```python
from build123d import *

# Parameters (mm, degrees)
F1_DEPTH = 10
F2_D     = 12
F2_DEPTH = 30


with BuildPart() as f1:
    # F0 (on Front) → F1 (new body)
    with BuildSketch(Plane.XZ):
        with BuildLine():
            ThreePointArc((0, -40), (8.838835, -36.338835), (12.5, -27.5))
            Line((12.5, -27.5), (12.5, 27.5))
            ThreePointArc((12.5, 27.5), (8.838835, 36.338835), (0, 40))
            ThreePointArc((0, 40), (-8.838835, 36.338835), (-12.5, 27.5))
            Line((-12.5, 27.5), (-12.5, -27.5))
            ThreePointArc((-12.5, -27.5), (-8.838835, -36.338835), (0, -40))
        make_face()
    extrude(amount=F1_DEPTH)

    # F2
    with Locations(Plane(origin=(0, 0, 0), x_dir=(1, 0, 0), z_dir=(0, 1, 0))):
        with Locations((0, 27.5), (0, -27.5)):
            Hole(F2_D / 2, depth=F2_DEPTH)


solid = f1.part
```
Could you check a few things on this model? Use its own coordinates, in mm. Coordinates: 2 decimals unless noted, no trailing zeros. Loops run counter-clockwise (first coordinate to the right, second up) from the corner with the lowest first, then second, coordinate; pieces in that order, holes last. Notation, with made-up numbers: M -28.5,57.5 L 25.5,57.5 A11 cw 25.5,69.5 Z; hole C 86,83.5 d4. An arc over 180 degrees is marked long. Put each result on its own line as item: value. Start each with the question number.
(1) I need wall thicknesses on line 1 (Z direction, x = 0, y = -3.25); line 2 (X direction, y = -6, z = -27.5); line 3 (Z direction, x = -1.5, y = -4.25). Which ranges of each line are inside material? Lowest first, please. Write a range as from..to.
(2) Suppose I cut it at A-A on z = -31.5. Please give me the cut outline in (x, y).
(3) Suppose I cut it at B-B on y = -8.5. Please give me the cut outline in (x, z), then the cut area to 3 significant figures.
(4) Will this pin go through, and if not, where does the flat tip stop? P1, Ø9.5, axis at x = 0, z = -27.5, coming from the +Y side.
(5) Suppose I cut it at C-C on x = -7. Please give me the cut outline in (y, z), then the cut area to 3 significant figures.
(6) Thinking about a two-plate mould opening in Z: for faces 1 (the face through (-12.5, -5, 0)), 2 (the face through (1.301, -5.07, -21.643)), which applies, pulls with the +Z half, pulls with the -Z half, needs draft (parallel to the pull), parting line crosses it, or undercut?
Solutions:
1. line 1: z = -40..-33.5, -21.5..21.5, 33.5..40
1. line 2: x = -12.5..-6, 6..12.5
1. line 3: z = -39.91..-33.31, -21.69..21.69, 33.31..39.91
2. outline: M -11.84,-10 L -4.47,-10 L -4.47,0 L -11.84,0 Z; M 4.47,-10 L 11.84,-10 L 11.84,0 L 4.47,0 Z
3. outline: M -12.5,-27.5 A12.5 ccw 0,-40 A12.5 ccw 12.5,-27.5 L 12.5,27.5 A12.5 ccw 0,40 A12.5 ccw -12.5,27.5 Z; hole C 0,-27.5 d12; hole C 0,27.5 d12
3. area: 1,640 mm2
4. P1: passes through
5. outline: M -10,-37.86 L 0,-37.86 L 0,37.86 L -10,37.86 Z
5. area: 757 mm2
6. face 1: needs draft
6. face 2: undercut
